Geometry: final body of the model. Coordinates: model frame, mm. A direction names the side the tool comes from. Coordinates: 2 decimals unless noted, no trailing zeros. Loops run counter-clockwise (first coordinate to the right, second up) from the corner with the lowest first, then second, coordinate; pieces in that order, holes last. Notation, with made-up numbers: (33.25, -33.5) - (68.25, -33.5) arc R15 cw to (68.25, -13.5) - close; hole circle Ø11 at (-8, -31.75). An arc over 180 degrees is marked (long way). Answer in a Markdown table with one row per item.
from build123d import *

# Parameters (mm, degrees)
ESQUISSE1_W             = 5
ESQUISSE1_H             = 175
ESQUISSE1_R             = 1
BOSS_EXTRU_1_DEPTH      = 80
ESQUISSE2_W             = 70
ESQUISSE2_H             = 15
ENL_V_MAT_EXTRU_1_DEPTH = 20


with BuildPart() as part:
    # Esquisse1 → Boss.-Extru.1 (new body)
    with BuildSketch(Plane.XY):
        with Locations((-4.901501369, 41.380516432)):
            Rectangle(ESQUISSE1_W, ESQUISSE1_H)
        with Locations((-4.956438342, 123.880516432)):
            Circle(ESQUISSE1_R, mode=Mode.SUBTRACT)
    extrude(amount=BOSS_EXTRU_1_DEPTH)

    # Esquisse2 → Enlèv. mat.-Extru.1 (cut)
    with BuildSketch(Plane(origin=(0, 0, 0), x_dir=(0, 0, -1), z_dir=(1, 0, 0))):
        with Locations((-40, 121.380516432)):
            Rectangle(ESQUISSE2_W, ESQUISSE2_H)
    extrude(amount=-ENL_V_MAT_EXTRU_1_DEPTH, mode=Mode.SUBTRACT)


solid = part.part
(1) First-contact query: pin 1 Ø1.2 at (x, y) = (-4.96, 123.88) entering from +Z; pin 2 Ø1.5 at (x, z) = (-4.5, 24.5) entering from +Y. Flat tips, straight axial feed; report the tip coordinate or a pass-through.
Verdict:
| item | result |
|---|---|
| pin 1 | passes through |
| pin 2 | stops at y = 113.88 |
(2) Cut plane C-C on z = 14. Output: boundary loops of the cut face in (x, y), then the cut area to 3 significant figures.
Verdict:
| item | result |
|---|---|
| outline | (-7.4, -46.12) - (-2.4, -46.12) - (-2.4, 113.88) - (-7.4, 113.88) - close |
| area | 800 mm² |
(3) Ray query, probe 1 along Z at (x, y) = (-3.35, 118.5); probe 2 along Y at (x, z) = (-4.6, 20). Return the intervals inside material, ascending.
Verdict:
| item | result |
|---|---|
| probe 1 | z = 0 to 5, 75 to 80 |
| probe 2 | y = -46.12 to 113.88 |
(4) Pull-direction query (Z, two-part tool) for faces 1 (the face through (-5, 128.881, 2)), 2 (the face through (-5, 113.881, 40)), 3 (the face through (-5, 43, 0)); classes: pulls with the +Z half, pulls with the -Z half, needs draft (parallel to the pull), parting line crosses it, or undercut.
Verdict:
| item | result |
|---|---|
| face 1 | needs draft |
| face 2 | undercut |
| face 3 | pulls with the -Z half |
(5) Access query for faces 4 (the face through (-5, 121, 5)), 5 (the face through (-5, 128.881, 77)). Directions: +Z, -Z, +X, -X, +Y, -Y. A direction counts if a zero-diameter tool reaches every point of the face in a straight line with its end or side. Return the directions, or none.
Verdict:
| item | result |
|---|---|
| face 4 | +X, -X, +Y |
| face 5 | +Z, -Z, +X, -X, +Y |
(6) Cut plane B-B on x = -3.2. Output: boundary loops of the cut face in (y, z), then the cut area to 4 significant figures.
Verdict:
| item | result |
|---|---|
| outline | (-46.12, 0) - (128.88, 0) - (128.88, 5) - (113.88, 5) - (113.88, 75) - (128.88, 75) - (128.88, 80) - (-46.12, 80) - close |
| area | 12,950 mm² |
(7) Cut plane A-A on y = 115.5. Output: boundary loops of the cut face in (x, z).
Verdict:
| item | result |
|---|---|
| outline | (-7.4, 0) - (-2.4, 0) - (-2.4, 5) - (-7.4, 5) - close; (-7.4, 75) - (-2.4, 75) - (-2.4, 80) - (-7.4, 80) - close |
